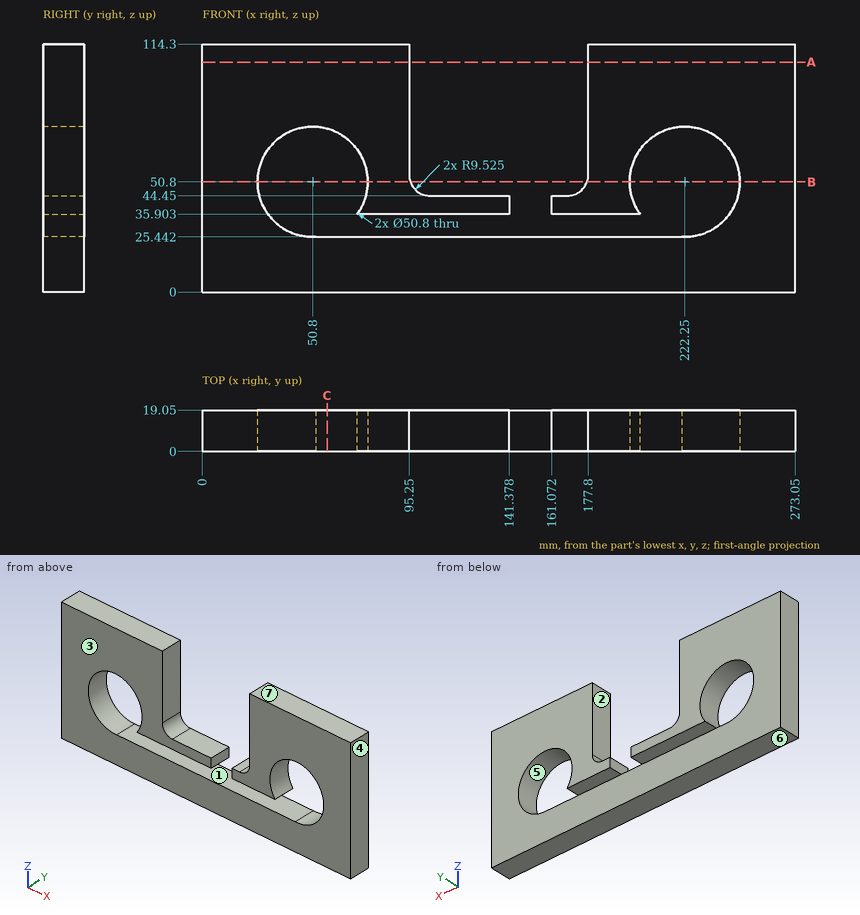
Here's the drawing with two shaded views (mm, measured from the low corner). I have some questions. A direction names the side the tool comes from. Round coordinates to 2 decimals unless told otherwise and drop trailing zeros. Loops run counter-clockwise (first coordinate to the right, second up) from the corner with the lowest first, then second, coordinate; pieces in that order, holes last. Notation, with made-up numbers: (75.25, -0.75) -> (87.25, -0.75) arc R6 cw to (87.25, 4.25) -> close; hole circle Ø4 at (-24, 38.25). An arc over 180 degrees is marked (long way). Answer as CSV lines item,"result". Start each with the question number.
1. Imagine slicing it at C-C on x = 57.5. Write out the boundary of the cut face in (y, z).
2. Imagine slicing it at B-B on z = 50.8. State how many separate pieces and enclosed holes the cut face has, plus the area to 3 significant figures.
3. I need wall thicknesses on probe 1 along X at (y, z) = (18, 41.5); probe 2 along Z at (x, y) = (222.25, 7.5); probe 3 along X at (y, z) = (13.75, 102.5). Which ranges of each line are inside material? Lowest first, please. Write a range as from..to.
4. Imagine slicing it at A-A on z = 106. Write out the boundary of the cut face in (x, y), plus the area to 3 significant figures.
5. If we mould it in two halves opening along Z, with no side actions, what happens to the marked faces 4, 5, 6 and 7? For each: pulls with the +Z half, pulls with the -Z half, needs draft (parallel to the pull), parting line crosses it, or undercut.
6. I'm going to push a flat-ended pin straight in: P1, Ø6, axis at x = 164, y = 5, coming from the +Z side. Where does the tip first touch, or does it pass through?
7. For the marked faces 1, 2 and 3, which set-ups out of +Z, -Z, +X, -X, +Y, -Y let a thin tool reach every point of the face, with its end or its side?
Solution:
1,outline,"(0, 0) -> (19.05, 0) -> (19.05, 25.44) -> (0, 25.44) -> close; (0, 75.3) -> (19.05, 75.3) -> (19.05, 114.3) -> (0, 114.3) -> close"
2,separate pieces,"4"
2,enclosed holes,"0"
2,area,"1,710 mm²"
3,probe 1,"0..27.16, 74.44..141.38, 161.07..198.61, 245.89..273.05"
3,probe 2,"0..25.4, 76.2..114.3"
3,probe 3,"0..95.25, 177.8..273.05"
4,outline,"(0, 0) -> (95.25, 0) -> (95.25, 19.05) -> (0, 19.05) -> close; (177.8, 0) -> (273.05, 0) -> (273.05, 19.05) -> (177.8, 19.05) -> close"
4,area,"3,630 mm²"
5,face 4,"needs draft"
5,face 5,"undercut"
5,face 6,"pulls with the -Z half"
5,face 7,"pulls with the +Z half"
6,P1,"z = 44.45"
7,face 1,"+Y, -Y"
7,face 2,"+Z, +Y, -Y"
7,face 3,"+Z, -Z, +X, -X, -Y"
